Autodesk Inventor part; units mm, degrees
ref_plane "作業平面1" through (7.1, 0, 14) normal (1, 0, 0) x (0, 0, -1)
ref_plane "作業平面2" through (-7.1, 0, 10.5) normal (1, 0, 0) x (0, 0, -1)
ref_plane "YZ Plane" through (0, 0, 0) normal (1, 0, 0) x (0, 1, 0)
sketch "スケッチ1" plane through (0, 0, 0) normal (0, 1, 0) x (-1, 0, 0)
  line L0 (4.6, 10.5) -> (-4.6, 10.5)
  line L1 (-4.6, 10.5) -> (-4.6, -10.5)
  line L2 (-4.6, -10.5) -> (4.6, -10.5)
  line L3 (4.6, -10.5) -> (4.6, 10.5)
  line L4 (4.6, -10.5) -> (-4.6, 10.5) construction
  line L5 (4.6, 10.5) -> (-4.6, -10.5) construction
  line L6 (9.6, 10.5) -> (9.6, -10.5)
  line L7 (-9.6, 10.5) -> (-9.6, -10.5)
  line L8 (0, 4) -> (0, -4) construction
  line L9 (0, 11.75) -> (0, -11.75) construction
  line L10 (9.6, -10.5) -> (9.6, -14)
  line L11 (9.6, -14) -> (-9.6, -14)
  line L12 (-9.6, -14) -> (-9.6, -10.5)
  line L13 (-9.6, 10.5) -> (-9.6, 14)
  line L14 (-9.6, 14) -> (9.6, 14)
  line L15 (9.6, 14) -> (9.6, 10.5)
  point P0 (0, 0)
  point P1 (0, 0)
  point P2 (0, 0)
  dimension "d0" = 21
  dimension "d1" = 9.2
  dimension "d2" = 5
  dimension "d3" = 23.5
  dimension "d4" = 8
  dimension "d21" = 3.5
  dimension "d26" = 5
  dimension "d27" = 3.5
extrude "押し出し1" add sketch "スケッチ1" along normal blind 2
hole "穴1" at (0, 0, 4) at (0, 0, -4) at (0, 0, 11.75) at (0, 0, -11.75) direction (0, 1, 0) diameter 1.5 end through all
sketch "スケッチ2" plane through (0, 2, 0) normal (0, 1, 0) x (1, 0, 0)
  line L0 (-4.6, -10.5) -> (-4.6, 10.5)
  circle A0 centre (0, -11.75) radius 0.75
  circle A1 centre (0, 11.75) radius 0.75
  line L1 (-9.6, 14) -> (-9.6, -14)
  line L2 (9.6, -14) -> (9.6, 14)
  line L3 (9.6, 14) -> (-9.6, 14)
  line L4 (-9.6, -14) -> (9.6, -14)
  line L5 (-9.6, 14) -> (-9.6, -14)
  line L6 (-9.6, -14) -> (9.6, -14)
  line L7 (-4.6, -14) -> (-9.6, -14)
  line L8 (-9.6, -14) -> (-9.6, -9)
  line L9 (-9.6, -9) -> (-4.6, -9)
  line L10 (-4.6, -9) -> (-4.6, -14)
  point P0 (0, 0)
  dimension "d28" = 5
extrude "押し出し2" add sketch "スケッチ2" along normal blind 5 contours L10 L4 L1 L9 L0
sketch "スケッチ6" plane through (-4.6, 2, 9) normal (0, 0, -1) x (-1, 0, 0)
  line L0 (5, 0) -> (0, 5) construction
  line L1 (5, 5) -> (0, 0) construction
  circle A0 centre (2.5, 2.5) radius 1.25
  point P0 (-4.6, -2)
  dimension "d29" = 2.5
extrude "押し出し5" cut sketch "スケッチ6" along normal through all both and the other way through all
mirror "ミラー4" about plane through (0, 0, 0) normal (0, 0, 1) of "押し出し2", "押し出し5"
sketch "スケッチ7" plane through (0, 2, 0) normal (0, 1, 0) x (1, 0, 0)
  line L0 (-4.6, 9) -> (-9.6, 9)
  line L1 (-9.6, -9) -> (-4.6, -9)
  line L2 (-4.6, -9) -> (-9.6, 9) construction
  line L3 (-4.6, 9) -> (-9.6, -9) construction
  line L4 (-6.1, -9) -> (-8.1, -9)
  line L5 (-8.1, -9) -> (-8.1, 9)
  line L6 (-8.1, 9) -> (-6.1, 9)
  line L7 (-6.1, 9) -> (-6.1, -9)
  line L8 (-6.1, -9) -> (-8.1, 9) construction
  point P0 (0, 0)
  point P1 (-7.1, 0)
  point P2 (-8.1, -9)
  dimension "d32" = 2
extrude "押し出し6" cut sketch "スケッチ7" against normal through all
mirror "ミラー5" about plane through (0, 0, 0) normal (1, 0, 0) of "押し出し2", "押し出し5", "ミラー4", "押し出し6"
fillet "フィレット1" radius 1.2 8 edges at (-8.85, 2, -9) (-5.35, 2, -9) (5.35, 2, -9) (8.85, 2, -9) (-8.85, 2, 9) (-5.35, 2, 9) (5.35, 2, 9) (8.85, 2, 9)
ref_plane "作業平面1" through (7.1, 0, 14) normal (1, 0, 0) x (0, 0, -1)
ref_plane "作業平面2" through (-7.1, 0, 10.5) normal (1, 0, 0) x (0, 0, -1)
equation "\"d26\" = d2"
equation "\"d27\" = d21"
properties part number "om_DropBase" material "ABS プラスチック"
The listing builds one solid part. Answer for the finished solid, in the listing's coordinates (mm). A direction names the side the tool comes from. Give positions to 0.01 mm unless a question says otherwise; leave off trailing zeros. Write each loop counter-clockwise with the first axis right and the second up, starting at its lowest first coordinate (ties: lowest second). Pieces come first, ordered by that corner, then holes. Notation, with made-up numbers: (6.25, -9.5) -> (54.25, -9.5) arc R7 ccw to (54.25, 2.5) -> close; hole circle Ø1 at (39.5, 47). An arc over 180 degrees is marked (long way). One line per question, with ' | ' between items. Start each with the question number.
1. Section D-D (y = 1.25) is taken. Determine the outline of the cut face in (x, z), plus the area to 3 significant figures.
2. For a pull along Y with two mould halves and no side action, classify faces 6 (the cylindrical face through (-6.83, 5.72, -11.46)), 7 (the flat face through (9, 2, 0)), 8 (the flat face through (8.2, 3.5, -9)) as pulls with the +Y half, pulls with the -Y half, needs draft (parallel to the pull), parting line crosses it, or undercut.
3. Find the intervals of material crossed by probe 1 along Z at (x, y) = (0, 1.45); probe 2 along Z at (x, y) = (7.5, 1.75); probe 3 along Y at (x, z) = (-7.1, 10.4), in increasing order.
4. Section C-C (x = 3.75) is taken. Determine the outline of the cut face in (y, z), plus the area to 3 significant figures.
5. For faces 1 (the flat face through (6.1, 1, 0)), 2 (the flat face through (-7, 7, 11)), 3 (the flat face through (0, 1, 14)), 4 (the cylindrical face through (8.84, 2.342, 8.639)), 5 (the flat face through (4.6, 1, 0)), determine the directions among +Z, -Z, +X, -X, +Y, -Y from which every point of the face is accessible in a straight line to the end or side of a thin tool.
6. Given pin 1 Ø4 at (x, y) = (4, 6) entering from +Z; pin 2 Ø1.6 at (x, z) = (9, -2) entering from +Y, each flat-ended and moving along its own axis, determine where each tip first touches the part or whether it passes through.
7. Section A-A (z = 11.75) is taken. Determine the outline of the cut face in (x, y), plus the area to 3 significant figures.
8. Section B-B (x = 7.1) is taken. Determine the outline of the cut face in (y, z), plus the area to 3 significant figures.
Response values:
1) outline: (-9.6, -14) -> (9.6, -14) -> (9.6, 14) -> (-9.6, 14) -> close; hole (-8.1, -9) -> (-6.1, -9) -> (-6.1, 9) -> (-8.1, 9) -> close; hole (-4.6, -10.5) -> (4.6, -10.5) -> (4.6, 10.5) -> (-4.6, 10.5) -> close; hole circle Ø1.5 at (0, -11.75); hole circle Ø1.5 at (0, 11.75); hole (6.1, -9) -> (8.1, -9) -> (8.1, 9) -> (6.1, 9) -> close | area: 269 mm2
2) face 6: undercut | face 7: pulls with the +Y half | face 8: needs draft
3) probe 1: -14 to -12.5, -11 to -10.5, 10.5 to 11, 12.5 to 14 | probe 2: -14 to -9, 9 to 14 | probe 3: 0 to 3.25, 5.75 to 7
4) outline: (0, -14) -> (2, -14) -> (2, -10.5) -> (0, -10.5) -> close; (0, 10.5) -> (2, 10.5) -> (2, 14) -> (0, 14) -> close | area: 14.0 mm2
5) face 1: +Y, -Y | face 2: +Z, -Z, +X, -X, +Y | face 3: +Z, +X, -X, +Y, -Y | face 4: +X, -X, +Y | face 5: +Y
6) pin 1: z = 14 | pin 2: y = 2
7) outline: (-9.6, 0) -> (-0.75, 0) -> (-0.75, 2) -> (-4.6, 2) -> (-4.6, 7) -> (-9.6, 7) -> close; (0.75, 0) -> (9.6, 0) -> (9.6, 7) -> (4.6, 7) -> (4.6, 2) -> (0.75, 2) -> close; hole circle Ø2.5 at (-7.1, 4.5); hole circle Ø2.5 at (7.1, 4.5) | area: 75.6 mm2
8) outline: (0, -14) -> (3.25, -14) -> (3.25, -9) -> (0, -9) -> close; (0, 9) -> (3.25, 9) -> (3.25, 14) -> (0, 14) -> close; (5.75, -14) -> (7, -14) -> (7, -9) -> (5.75, -9) -> close; (5.75, 9) -> (7, 9) -> (7, 14) -> (5.75, 14) -> close | area: 45.0 mm2
